Drawing for the job (mm, zero at the part's lowest x, y, z). Coordinates: 2 decimals unless noted, no trailing zeros. Loops run counter-clockwise (first coordinate to the right, second up) from the corner with the lowest first, then second, coordinate; pieces in that order, holes last.
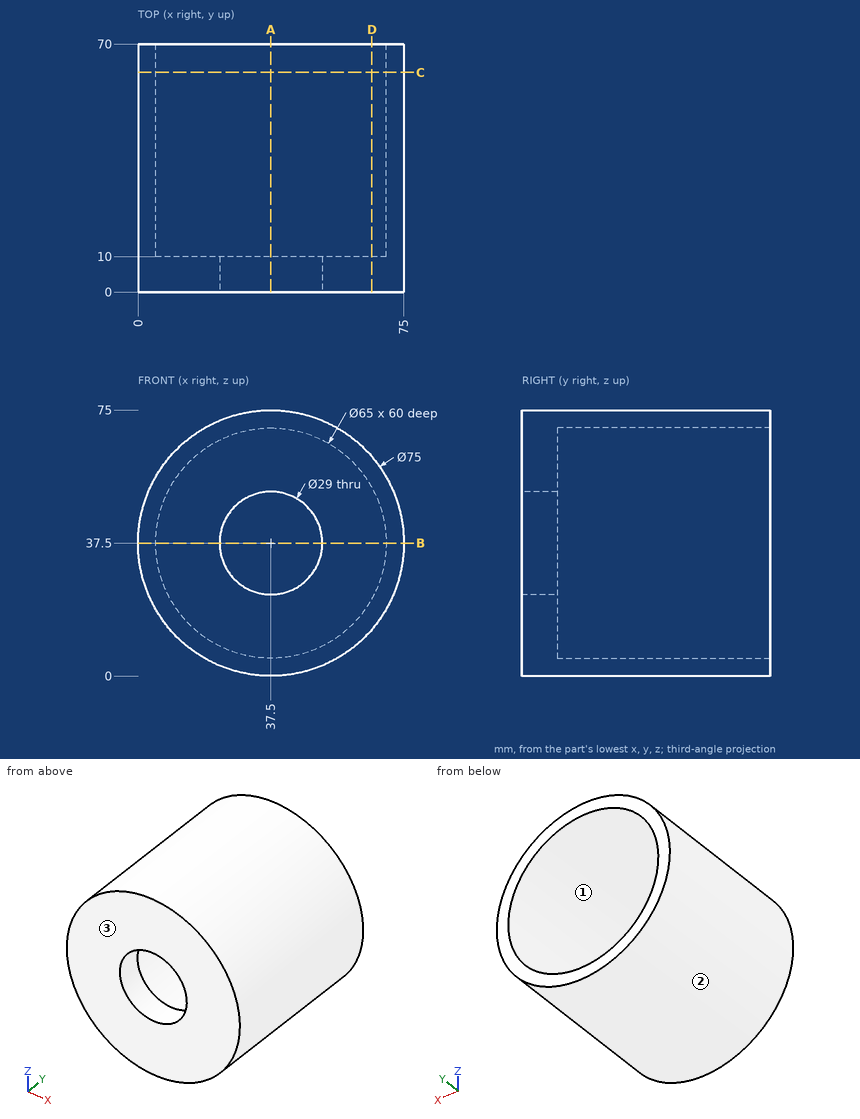
Q1. Saw through at B-B (z = 37.5). List the corners of the cut face in (x, y), plus the area to 3 significant figures.
Q2. Probe line 1 (X direction, y = 39.5, z = 37.5); line 2 (X direction, y = 5.5, z = 37.5). List the from-to ranges inside material, lowest first.
Q3. Saw through at D-D (x = 66). List the corners of the cut face in (y, z), plus the area to 3 significant figures.
Q4. Saw through at A-A (x = 37.5). List the corners of the cut face in (y, z), plus the area to 3 significant figures.
Q5. Drop flat-ended pins along their axis: P1, Ø6, axis at y = 43, z = 63.5, coming from the +X side; P2, Ø1.5, axis at y = 29, z = 38.5, coming from the +X side; P3, Ø3, axis at x = 43, y = 11, coming from the +Z side. Give the stop position or say it passes through.
Q6. Mould opens along X. For the marked faces 1, 2 and 3 say: released by +X, released by -X, zero draft, split by the parting line, or undercut.
Q7. Saw through at C-C (y = 62). List the corners of the cut face in (x, z).
Checked values:
1. outline: (0, 0) - (23, 0) - (23, 10) - (5, 10) - (5, 70) - (0, 70) - close; (52, 0) - (75, 0) - (75, 70) - (70, 70) - (70, 10) - (52, 10) - close
1. area: 1,060 mm2
2. line 1: x = 0 to 5, 70 to 75
2. line 2: x = 0 to 23, 52 to 75
3. outline: (0, 13.13) - (70, 13.13) - (70, 21.88) - (10, 21.88) - (10, 53.12) - (70, 53.12) - (70, 61.87) - (0, 61.87) - close
3. area: 1,540 mm2
4. outline: (0, 0) - (70, 0) - (70, 5) - (10, 5) - (10, 23) - (0, 23) - close; (0, 52) - (10, 52) - (10, 70) - (70, 70) - (70, 75) - (0, 75) - close
4. area: 1,060 mm2
5. P1: stops at x = 67.12
5. P2: stops at x = 75
5. P3: stops at z = 74.79
6. face 1: undercut
6. face 2: split by the parting line
6. face 3: zero draft
7. outline: circle Ø75 at (37.5, 37.5); hole circle Ø65 at (37.5, 37.5)
